The listing builds one solid part. Answer for the finished solid, in the listing's coordinates (mm). A direction names the side the tool comes from. Give positions to 0.01 mm unless a question says otherwise; leave off trailing zeros. Order: outer loops, then holes, each group sorted by start corner. A loop starts at its lowest first (then second) coordinate and runs counter-clockwise, first axis right, second up.
Autodesk Inventor part; units mm, degrees
ref_plane "Work Plane1" through (41.411, -174.5481, 0) normal (0, -1, 0) x (1, 0, 0)
ref_plane "YZ Plane" through (0, 0, 0) normal (1, 0, 0) x (0, 1, 0)
ref_plane "XZ Plane" through (0, 0, 0) normal (0, 1, 0) x (-1, 0, 0)
sketch "Sketch1" plane through (0, 0, 0) normal (0, 0, 1) x (1, 0, 0)
  line L0 (0, 0) -> (160, 0) construction
  line L1 (160, 0) -> (118.589, -154.5481) construction
  line L2 (0, 0) -> (41.411, -154.5481) construction
  line L3 (41.411, -154.5481) -> (118.589, -154.5481)
  circle A0 centre (235.8871, -103.156) radius 80 construction
  line L4 (160, 0) -> (256.5926, -25.8819)
  line L5 (118.589, -154.5481) -> (215.1815, -180.43)
  arc A1 (215.1815, -180.43) -> (256.5926, -25.8819) centre (235.8871, -103.156) ccw
  circle A2 centre (-75.8871, -103.156) radius 80 construction
  line L6 (0, 0) -> (-96.5926, -25.8819)
  line L7 (41.411, -154.5481) -> (-55.1815, -180.43)
  arc A3 (-96.5926, -25.8819) -> (-55.1815, -180.43) centre (-75.8871, -103.156) ccw
  arc A4 (160, 0) -> (0, 0) centre (80, -304.672) ccw
  dimension "d0" = 160
  dimension "d1" = 160
  dimension "d2" = 160
  dimension "d3" = 75
  dimension "d4" = 75
  dimension "d5" = 160
  dimension "d6" = 100
  dimension "d7" = 160
  dimension "d9" = 100
  dimension "d56" = 315
extrude "Extrusion1" add sketch "Sketch1" along normal blind 41.5
sketch "Sketch2" plane through (0, 0, 41.5) normal (0, 0, 1) x (1, 0, 0)
  line L0 (-26.5, -133) -> (186.5, -133)
  line L1 (186.5, -133) -> (186.5, -20)
  line L2 (186.5, -20) -> (-26.5, -20)
  line L3 (-26.5, -20) -> (-26.5, -133)
  line L4 (0, 0) -> (-96.5926, -25.8819)
  arc A0 (160, 0) -> (0, 0) centre (80, -304.672) ccw
  line L5 (0, 0) -> (160, 0)
  point P0 (80, -20)
  point P1 (80, 0)
  dimension "d12" = 213
  dimension "d13" = 113
  dimension "d57" = 20
extrude "Extrusion2" cut sketch "Sketch2" against normal through all contours L3 L2 L1 L0
sketch "Sketch3" plane through (0, 0, 41.5) normal (0, 0, 1) x (1, 0, 0)
  line L0 (186.5, -20) -> (186.5, -133) construction
  line L1 (186.5, -133) -> (-26.5, -133) construction
  line L2 (-26.5, -133) -> (-26.5, -20) construction
  line L3 (-26.5, -20) -> (186.5, -20) construction
  line L4 (0, 0) -> (-96.5926, -25.8819) construction
  arc A0 (-96.5926, -25.8819) -> (-55.1815, -180.43) centre (-75.8871, -103.156) ccw construction
  line L5 (-55.1815, -180.43) -> (41.411, -154.5481) construction
  line L6 (41.411, -154.5481) -> (118.589, -154.5481) construction
  line L7 (118.589, -154.5481) -> (215.1815, -180.43) construction
  arc A1 (215.1815, -180.43) -> (256.5926, -25.8819) centre (235.8871, -103.156) ccw construction
  line L8 (256.5926, -25.8819) -> (160, 0) construction
  line L9 (-48.0481, -154.5481) -> (208.0481, -154.5481) construction
  line L10 (208.0481, -154.5481) -> (208.0481, 10.328) construction
  line L11 (-48.0481, 10.328) -> (-48.0481, -154.5481) construction
  line L12 (-48.0481, 10.328) -> (-48.0481, -178.5186)
  line L13 (-55.1815, -180.43) -> (41.411, -154.5481)
  line L14 (208.0481, 10.328) -> (208.0481, -178.5186)
  line L15 (118.589, -154.5481) -> (215.1815, -180.43)
  line L16 (-48.0481, -178.5186) -> (208.0481, -178.5186)
  line L17 (-48.0481, 10.328) -> (208.0481, 10.328)
  line L18 (-157.6505, -218.8456) -> (317.6505, -218.8456)
  line L19 (317.6505, -218.8456) -> (317.6505, 50.655)
  line L20 (317.6505, 50.655) -> (-157.6505, 50.655)
  line L21 (-157.6505, 50.655) -> (-157.6505, -218.8456)
  arc A2 (160, 0) -> (0, 0) centre (80, -304.672) ccw
  point P0 (80, -154.5481)
  point P1 (80, 10.328)
  point P2 (208.0481, -84.0953)
  point P3 (317.6505, -84.0953)
  point P4 (80, 10.328)
  point P5 (80, -218.8456)
  dimension "d22" = 269.5006
  dimension "d23" = 475.3011
extrude "Extrusion3" cut sketch "Sketch3" against normal through all
sketch "Sketch5" plane through (0, 0, 41.5) normal (0, 0, 1) x (1, 0, 0)
  line L0 (118.589, -154.5481) -> (208.0481, -178.5186)
  line L1 (208.0481, -178.5186) -> (80, -178.5186)
  line L2 (80, -178.5186) -> (80, 10.328)
  line L3 (80, 10.328) -> (208.0481, 10.328)
  line L4 (208.0481, 10.328) -> (208.0481, -178.5186)
  arc A0 (160, 0) -> (0, 0) centre (80, -304.672) ccw
extrude "Extrusion4" cut sketch "Sketch5" against normal through all
sketch "Sketch6" plane through (0, 0, 0) normal (0, 1, 0) x (-1, 0, 0)
  circle A0 centre (17, 20.75) radius 2
  line L0 (26.5, 41.5) -> (26.5, 0)
  point P0 (26.5, 20.75)
  dimension "d24" = 4
  dimension "d58" = 9.5
extrude "Extrusion5" cut sketch "Sketch6" along normal through all both and the other way through all
sketch "Sketch7" plane through (0, 0, 0) normal (0, 1, 0) x (-1, 0, 0)
  circle A0 centre (17, 20.75) radius 2
  circle A1 centre (17, 20.75) radius 6.5
  dimension "d59" = 13
extrude "Extrusion6" cut sketch "Sketch7" against normal blind 10
ref_plane "Work Plane1" through (41.411, -174.5481, 0) normal (0, -1, 0) x (1, 0, 0)
sketch "Sketch8" plane through (41.411, -174.5481, 0) normal (0, -1, 0) x (1, 0, 0)
  circle A0 centre (-58.411, 20.75) radius 2
  circle A1 centre (-58.411, 20.75) radius 6.5
  point P0 (-41.411, 0)
  dimension "d32" = 13
extrude "Extrusion7" cut sketch "Sketch8" against normal blind 10
sketch "Sketch11" plane through (41.411, -154.5481, 0) normal (0, -1, 0) x (1, 0, 0)
  line L0 (0, 41.5) -> (38.589, 41.5)
  line L1 (0, 0) -> (0, 41.5)
  line L2 (0, 0) -> (38.589, 0)
  line L3 (38.589, 0) -> (38.589, 41.5)
  circle A0 centre (19.2945, 20.75) radius 2.5
  circle A1 centre (19.2945, 20.75) radius 6.5
  point P0 (-41.411, 0)
  point P1 (0, 20.75)
  point P2 (19.2945, 41.5)
  dimension "d73" = 5
  dimension "d74" = 13
extrude "Extrusion10" cut sketch "Sketch11" against normal blind 10 contours A1
sketch "Sketch12" plane through (-48.0481, -178.5186, 41.5) normal (-1, 0, 0) x (0, 0, 1)
  line L0 (-41.5, 0) -> (-41.5, 165.6442)
  line L1 (0, 0) -> (-41.5, 0)
  line L2 (0, 165.6442) -> (0, 0)
  line L3 (-41.5, 165.6442) -> (0, 165.6442)
  line L4 (-5, 5) -> (-36.5, 5)
  line L5 (-36.5, 5) -> (-36.5, 160.6442)
  line L6 (-36.5, 160.6442) -> (-5, 160.6442)
  line L7 (-5, 160.6442) -> (-5, 5)
  point P0 (-41.5, 178.5186)
  dimension "d43" = 5
extrude "Extrusion11" cut sketch "Sketch12" against normal blind 15 contours L4 L5 L6 L7
sketch "Sketch13" plane through (0, 0, 41.5) normal (0, 0, 1) x (1, 0, 0)
  circle A0 centre (-40.0481, -95.6966) radius 2.5
  line L0 (-48.0481, -12.8745) -> (-48.0481, -178.5186)
  point P0 (0, 0)
  point P1 (-48.0481, -95.6966)
  dimension "d46" = 5
  dimension "d47" = 8
extrude "Extrusion12" cut sketch "Sketch13" against normal through all
sketch "Sketch14" plane through (0, 0, 41.5) normal (0, 0, 1) x (1, 0, 0)
  circle A0 centre (-40.0481, -95.6966) radius 2.5
  circle A1 centre (-40.0481, -95.6966) radius 6.5
  point P0 (0, 0)
  dimension "d50" = 13
extrude "Extrusion13" cut sketch "Sketch14" against normal blind 4
sketch "Sketch15" plane through (0, 0, 0) normal (0, 0, -1) x (-1, 0, 0)
  circle A0 centre (40.0481, -95.6966) radius 2.5
  circle A1 centre (40.0481, -95.6966) radius 2.5
  circle A2 centre (40.0481, -95.6966) radius 6.5
  point P0 (0, 0)
  dimension "d53" = 13
extrude "Extrusion14" cut sketch "Sketch15" against normal blind 4
sketch "Sketch16" plane through (0, 0, 41.5) normal (0, 0, 1) x (1, 0, 0)
  line L0 (80, -20) -> (80, 10.328) construction
  circle A0 centre (80, -4.836) radius 7 construction
  circle A1 centre (80, -4.836) radius 15.164 construction
  arc A2 (80, -20) -> (80, 10.328) centre (80, -4.836) ccw
  arc A3 (80, -11.836) -> (80, 2.164) centre (80, -4.836) ccw
  arc A4 (80, 10.328) -> (0, 0) centre (80, -304.672) ccw
  line L1 (80, 10.328) -> (80, 2.164)
  line L2 (80, -11.836) -> (80, -20)
  dimension "d62" = 14
extrude "Extrusion15" add sketch "Sketch16" against normal blind 41.5
sketch "Sketch17" plane through (0, 0, 41.5) normal (0, 0, 1) x (1, 0, 0)
  arc A0 (80, -11.836) -> (80, 2.164) centre (80, -4.836) ccw construction
  circle A1 centre (80, -4.836) radius 7
  point P0 (0, 0)
extrude "Extrusion16" cut sketch "Sketch17" against normal through all
sketch "Sketch19" plane through (0, 0, 41.5) normal (0, 0, 1) x (1, 0, 0)
  circle A0 centre (80, -4.836) radius 7
  arc A1 (80, -20) -> (80, 10.328) centre (80, -4.836) ccw
  circle A2 centre (80, -4.836) radius 15.164 construction
  circle A3 centre (80, -4.836) radius 16.164
  point P0 (0, 0)
  dimension "d72" = 1
extrude "Extrusion18" cut sketch "Sketch19" against normal blind 20.75
sketch "Sketch20" plane through (60.7055, -154.5481, 20.75) normal (0, -1, 0) x (1, 0, 0)
  circle A0 centre (0, 0) radius 2.5
  point P0 (-60.7055, -20.75)
extrude "Extrusion19" cut sketch "Sketch20" against normal blind 50
properties part number "Riser Base" material "ABS Plastic"
1) For a pull along Z with two mould halves and no side action, classify faces 1 (the flat face through (-23.688, -6.347, 20.46)), 2 (the flat face through (-41, -173.519, 21)), 3 (the flat face through (-28, -83, 41.5)) as +Z half, -Z half, draft (parallel to the pull), parting line (faces both ways), or undercut.
Geometry says:
face 1: draft
face 2: undercut
face 3: +Z half
2) Find section D-D (z = 34). Write down the section's boundary in (x, y).
Geometry says:
outline: (-48.05, -178.52) - (41.41, -154.55) - (80, -154.55) - (80, -133) - (-26.5, -133) - (-26.5, -20) - (74.4, -20) arc R16.16 cw to (74.26, 10.28) arc R315 ccw to (0, 0) - (-48.05, -12.87) - (-48.05, -17.87) - (-33.05, -17.87) - (-33.05, -173.52) - (-48.05, -173.52) - close
3) Find section C-C (x = 31). Write down the section's boundary in (y, z), then the cut area to 3 significant figures.
Geometry says:
outline: (-157.34, 0) - (-133, 0) - (-133, 41.5) - (-157.34, 41.5) - close; (-20, 0) - (6.49, 0) - (6.49, 41.5) - (-20, 41.5) - close
area: 2,110 mm2
4) Straight lines are drawn through the part: probe 1 along Z at (x, y) = (-17, -166); probe 2 along Z at (x, y) = (-17, -153); probe 3 along X at (y, z) = (-137, 20). For each, find the intervals that lie inside material, in ascending order.
Geometry says:
probe 1: z = 0 to 14.25, 27.25 to 41.5
probe 2: z = 0 to 18.75, 22.75 to 41.5
probe 3: x = -33.05 to -18.85, -15.15 to 58.32, 63.09 to 80
5) Find section A-A (y = -128). Write down the section's boundary in (x, z).
Geometry says:
outline: (-48.05, 0) - (-26.5, 0) - (-26.5, 41.5) - (-48.05, 41.5) - (-48.05, 36.5) - (-33.05, 36.5) - (-33.05, 5) - (-48.05, 5) - close
6) A tool of negligible diameter and unlimited length cuts with its end or side. For faces 4 (the cylindrical face through (-10.506, -7.145, 21.036)), 5 (the flat face through (56, -154.548, 16)), 6 (the cylindrical face through (66.905, -149.618, 22.702)), from which of +Z, -Z, +X, -X, +Y, -Y can it reach the whole face along a straight path? Write none if from no direction.
Geometry says:
face 4: +Y
face 5: +Z, -Z, +X, -Y
face 6: -Y
7) Given P1, Ø5, axis at x = -25, z = 24, coming from the +Y side; P2, Ø6.5, axis at x = -39, y = -93, coming from the +Z side; P3, Ø3, axis at x = -40.05, y = -95.7, coming from the +Z side; P4, Ø6.5, axis at x = 64, z = 20, coming from the -Y side, each flat-ended and moving along its own axis, determine where each tip first touches the part or whether it passes through.
Geometry says:
P1: stops at y = -6.03
P2: stops at z = 37.5
P3: passes through
P4: stops at y = -154.55
8) Find section B-B (x = -17). Write down the section's boundary in (y, z), then the cut area to 3 significant figures.
Geometry says:
outline: (-170.2, 0) - (-133, 0) - (-133, 18.75) - (-164.55, 18.75) - (-164.55, 14.25) - (-170.2, 14.25) - close; (-170.2, 27.25) - (-164.55, 27.25) - (-164.55, 22.75) - (-133, 22.75) - (-133, 41.5) - (-170.2, 41.5) - close; (-20, 0) - (-4.56, 0) - (-4.56, 14.25) - (-10, 14.25) - (-10, 18.75) - (-20, 18.75) - close; (-20, 22.75) - (-10, 22.75) - (-10, 27.25) - (-4.56, 27.25) - (-4.56, 41.5) - (-20, 41.5) - close
area: 1,870 mm2
